Input: part model. Units: mm. Frame: model coordinates. A direction names the side the tool comes from. Coordinates: 2 decimals unless noted, no trailing zeros. Loops run counter-clockwise (first coordinate to the right, second up) from the corner with the lowest first, then second, coordinate; pieces in that order, holes last. Notation, with made-up numbers: M 8,54 L 22,54 A33 cw 22,83 Z; hole C -23.5,89 d3. An arc over 180 degrees is marked long. Use a Markdown table: item, result. Add a question column.
1. Section B-B on x = -3.5. Output: boundary loops of the cut face in (y, z), then the cut area to 3 significant figures.
2. Draft query along X for faces 1 (the cylindrical face through (-9.43, 15.4, -24.53)), 2 (the flat face through (-5.147, 9.09, -23.486)), 3 (the flat face through (10, 2.8, -8.3)). Return one class per face: +X half, -X half, draft (parallel to the pull), parting line (faces both ways), or undercut.
3. Line query: L1, parallel to Z at x = 0, y = 1.8; L2, parallel to Z at x = 1.75, y = 12.25; L3, parallel to Y at x = 3.25, z = 8.5. Output: solid intervals per line, ascending. Write a range as [from, to].
4. Section C-C on y = 11. Output: boundary loops of the cut face in (x, z), then the cut area to 3 significant figures.
5. Pin query (flat end, axial travel): pin 1 (5 mm diameter, centred on x = 0, z = 15.5, fed in from -Y); pin 2 (3 mm diameter, centred on x = -7, y = 8, fed in from +Z); pin 3 (6 mm diameter, centred on x = -2.5, z = 2, fed in from +Y); pin 4 (4.5 mm diameter, centred on x = 2, y = 8.5, fed in from +Z). Return the tip coordinate at first contact, or that it passes through.
6. Section D-D on z = 3.5. Output: boundary loops of the cut face in (x, y), then the cut area to 3 significant figures.
7. Section A-A on z = -4.5. Output: boundary loops of the cut face in (x, y).
8. Set-up query: faces 4 (the flat face through (0, 11, -22.5)), 5 (the cylindrical face through (9.43, 15.4, -24.47)), 6 (the flat face through (2, 10.15, -23)). Return all of +Z, -Z, +X, -X, +Y, -Y with unobstructed straight access to the full face (end or side cutting, diameter ignored); none if empty.
Autodesk Inventor part; units mm, degrees
ref_plane "YZ Plane" through (0, 0, 0) normal (1, 0, 0) x (0, 1, 0)
ref_plane "XZ Plane" through (0, 0, 0) normal (0, 1, 0) x (-1, 0, 0)
ref_plane "XY Plane" through (0, 0, 0) normal (0, 0, 1) x (1, 0, 0)
sketch "Boceto1" plane through (0, 0, 0) normal (0, 1, 0) x (-1, 0, 0)
  line L0 (-10, 22.5) -> (10, 22.5)
  line L1 (10, 22.5) -> (10, -22.5)
  line L2 (10, -22.5) -> (-10, -22.5)
  line L3 (-10, -22.5) -> (-10, 22.5)
  line L4 (-10, 22.5) -> (10, -22.5) construction
  line L5 (10, 22.5) -> (-10, -22.5) construction
  circle A0 centre (0, 15.5) radius 2.7
  circle A1 centre (0, -4.5) radius 2.7
  point P0 (0, 0)
  point P1 (0, 0)
  dimension "d0" = 5.4
  dimension "d1" = 5.4
  dimension "d2" = 45
  dimension "d3" = 20
  dimension "d21" = 20
  dimension "d22" = 7
extrude "Extrusión1" add sketch "Boceto1" along normal blind 3
sketch "Boceto2" plane through (0, 0, 0) normal (0, -1, 0) x (1, 0, 0)
  line L0 (10, -22.5) -> (-10, -22.5)
  line L1 (10, -22.5) -> (-10, -22.5)
  line L2 (-10, -22.5) -> (-10, -26.5)
  line L3 (-10, -26.5) -> (10, -26.5)
  line L4 (10, -26.5) -> (10, -22.5)
  line L5 (-10, -22.5) -> (-10, 22.5)
  point P0 (0, 0)
  dimension "d8" = 4
extrude "Extrusión2" add sketch "Boceto2" against normal blind 16
sketch "Boceto3" plane through (10, 0, -26.5) normal (0, 0, -1) x (-1, 0, 0)
  circle A0 centre (7.5, 8) radius 1.2
  circle A1 centre (17, 8) radius 1.2
  line L0 (20, 0) -> (20, 16)
  line L1 (0, 16) -> (20, 16)
  point P0 (10, 0)
  dimension "d11" = 9.5
  dimension "d12" = 2.4
  dimension "d13" = 3
  dimension "d16" = 8
extrude "Extrusión3" cut sketch "Boceto3" against normal blind 20
sketch "Boceto4" plane through (-10, 3, -22.5) normal (0, 0, 1) x (1, 0, 0)
  circle A0 centre (12.5, 5) radius 1.2
  line L0 (14.9826, 5) -> (13.7413, 2.85)
  line L1 (13.7413, 2.85) -> (11.2587, 2.85)
  line L2 (11.2587, 2.85) -> (10.0174, 5)
  line L3 (10.0174, 5) -> (11.2587, 7.15)
  line L4 (11.2587, 7.15) -> (13.7413, 7.15)
  line L5 (13.7413, 7.15) -> (14.9826, 5)
  circle A1 centre (3, 5) radius 1.2
  line L6 (5.4826, 5) -> (4.2413, 2.85)
  line L7 (4.2413, 2.85) -> (1.7587, 2.85)
  line L8 (1.7587, 2.85) -> (0.5174, 5)
  line L9 (0.5174, 5) -> (1.7587, 7.15)
  line L10 (1.7587, 7.15) -> (4.2413, 7.15)
  line L11 (4.2413, 7.15) -> (5.4826, 5)
  circle A2 centre (12.5, 5) radius 2.15
  circle A3 centre (3, 5) radius 2.15
  point P0 (10, -3)
  dimension "d17" = 4.3
extrude "Extrusión4" cut sketch "Boceto4" against normal blind 2 contours A0 | L0 A2 L5 | L0 L1 A2 | A2 | A2 L4 L5 | L1 L2 A2 | A2 L3 L4 | L2 L3 A2 | A1 | L6 A3 L11 | L6 L7 A3 | A3 | A3 L10 L11 | L7 L8 A3 | A3 L9 L10 | L8 L9 A3
fillet "Empalme1" radius 2 2 edges at (-10, 1.5, 22.5) (10, 1.5, 22.5)
fillet "Empalme2" radius 2 2 edges at (-10, 16, -24.5) (10, 16, -24.5)
fillet "Empalme3" radius 2 1 edges at (0, 0, -26.5)
fillet "Empalme4" radius 4 1 edges at (0, 3, -22.5)
properties part number "zupportenstop"
Answers below:
| question | item | result |
|---|---|---|
| 1 | outline | M 0,-24.5 A2 ccw 2,-26.5 L 16,-26.5 L 16,-22.5 L 7,-22.5 A4 cw 3,-18.5 L 3,22.5 L 0,22.5 Z |
| 1 | area | 202 mm² |
| 2 | face 1 | -X half |
| 2 | face 2 | undercut |
| 2 | face 3 | +X half |
| 3 | L1 | z = [-26.49, -7.2], [-1.8, 12.8], [18.2, 22.5] |
| 3 | L2 | z = [-26.5, -22.5] |
| 3 | L3 | y = [0, 3] |
| 4 | outline | M -10,-26.5 L 10,-26.5 L 10,-22.5 L -10,-22.5 Z |
| 4 | area | 80.0 mm² |
| 5 | pin 1 | passes through |
| 5 | pin 2 | stops at z = -24.5 |
| 5 | pin 3 | stops at y = 3 |
| 5 | pin 4 | stops at z = -22.48 |
| 6 | outline | M -10,0 L 10,0 L 10,3 L -10,3 Z |
| 6 | area | 60.0 mm² |
| 7 | outline | M -10,0 L -2.7,0 L -2.7,3 L -10,3 Z; M 2.7,0 L 10,0 L 10,3 L 2.7,3 Z |
| 8 | face 4 | +Z, +X, -X, +Y |
| 8 | face 5 | +Z, -Z, +X, +Y |
| 8 | face 6 | +Z |
